Part model, mm, in its own coordinate system. Face numbers are marked on the shaded views. A direction names the side the tool comes from. Coordinates: 2 decimals unless noted, no trailing zeros. Write each loop counter-clockwise with the first axis right and the second up, starting at its lowest first coordinate (ties: lowest second). Pieces come first, ordered by that corner, then holes. Notation, with made-up numbers: M 24.5,-12.5 L 83.5,-12.5 A17 ccw 83.5,17.5 Z; hole C -23,22.25 d4. An arc over 180 degrees is marked long. Use a Markdown table: item, result. Add a question column.
Q1. Slice it at C-C on x = 0. Write the cut outline in (y, z), then the cut area to 3 significant figures.
Q2. Pin check, flat tips, straight feed: pin 1 Ø2.5 at (x, z) = (-2.5, -4) entering from +Y; pin 2 Ø2 at (y, z) = (20, 0) entering from -X; pin 3 Ø1 at (x, z) = (0.5, 0.5) entering from -Y; pin 4 Ø1.5 at (x, y) = (1, 17.5) entering from +Z. Stop position of each tip, or through.
Q3. Slice it at B-B on z = 0. Write the cut outline in (x, y).
Q4. Wall check: L1, parallel to Z at x = 1, y = 8.75; L2, parallel to Y at x = 1.5, z = -1.5; L3, parallel to Y at x = -2, z = 3.5. Give the ranges that are in metal, low to high. Write a range as from..to.
Q5. Slice it at D-D on y = 25. Write the cut outline in (x, z).
Q6. Tool access for the marked faces 1 and 2: list every direction of +Z, -Z, +X, -X, +Y, -Y with a clear straight run to the whole face (end or side of a thin tool).
Q7. Slice it at A-A on y = 4. Write the cut outline in (x, z), then the cut area to 3 significant figures.
Q8. Mould opens along Z. For the marked faces 3, 4, 5 and 6 say: released by +Z, released by -Z, zero draft, split by the parting line, or undercut.
Autodesk Inventor part; units mm, degrees
ref_plane "YZ Plane" through (0, 0, 0) normal (1, 0, 0) x (0, 1, 0)
ref_plane "XZ Plane" through (0, 0, 0) normal (0, 1, 0) x (-1, 0, 0)
ref_plane "XY Plane" through (0, 0, 0) normal (0, 0, 1) x (1, 0, 0)
sketch "Szkic1" plane through (0, 0, 0) normal (0, 1, 0) x (-1, 0, 0)
  line L0 (-2.75, 2.75) -> (2.75, 2.75)
  line L1 (2.75, 2.75) -> (2.75, -2.75)
  line L2 (2.75, -2.75) -> (-2.75, -2.75)
  line L3 (-2.75, -2.75) -> (-2.75, 2.75)
  line L4 (-2.75, 2.75) -> (2.75, -2.75) construction
  line L5 (2.75, 2.75) -> (-2.75, -2.75) construction
  line L6 (-2, 6) -> (2, 6)
  line L7 (6, 2) -> (6, -2)
  line L8 (2, -6) -> (-2, -6)
  line L9 (-6, -2) -> (-6, 2)
  line L10 (-6, 6) -> (6, -6) construction
  line L11 (6, 6) -> (-6, -6) construction
  arc A0 (6, 2) -> (2, 6) centre (2, 2) ccw
  arc A1 (2, -6) -> (6, -2) centre (2, -2) ccw
  arc A2 (-6, -2) -> (-2, -6) centre (-2, -2) ccw
  arc A3 (-2, 6) -> (-6, 2) centre (-2, 2) ccw
  point P0 (0, 0)
  dimension "d0" = 5.5
  dimension "d1" = 12
  dimension "d2" = 4
extrude "Wyciągnięcie proste1" add sketch "Szkic1" along normal blind 10
sketch "Szkic2" plane through (0, 10, 0) normal (0, 1, 0) x (1, 0, 0)
  arc A0 (-6, -2) -> (-2, -6) centre (-2, -2) ccw
  line L0 (-6, 2) -> (-6, -2)
  arc A1 (-2, 6) -> (-6, 2) centre (-2, 2) ccw
  line L1 (2, 6) -> (-2, 6)
  arc A2 (6, 2) -> (2, 6) centre (2, 2) ccw
  line L2 (6, -2) -> (6, 2)
  arc A3 (2, -6) -> (6, -2) centre (2, -2) ccw
  line L3 (-2, -6) -> (2, -6)
extrude "Wyciągnięcie proste2" add sketch "Szkic2" along normal blind 2
sketch "Szkic3" plane through (0, 12, 0) normal (0, 1, 0) x (1, 0, 0)
  circle A0 centre (0, 0) radius 4
  dimension "d7" = 8
extrude "Wyciągnięcie proste3" add sketch "Szkic3" along normal blind 15.45
sketch "Szkic5" plane through (0, 12, 0) normal (0, 1, 0) x (1, 0, 0)
  circle A0 centre (0, 0) radius 5.1
  dimension "d19" = 10.2
extrude "Wyciągnięcie proste4" add sketch "Szkic5" along normal blind 6.15
fillet "Zaokrąglenie2" radius 0.25 1 edges at (-4, 27.45, 0)
chamfer "Faza1" distance 1 angle 45 4 edges at (-2.75, 10, 0) (0, 10, 2.75) (2.75, 10, 0) (0, 10, -2.75)
sketch "Sketch6" plane through (0, 18.15, 0) normal (0, 1, 0) x (1, 0, 0)
  circle A0 centre (0, 0) radius 5.1
  circle A1 centre (0, 0) radius 4
extrude "Extrusion5" add sketch "Sketch6" along normal blind 3.3 contours A0 | A1
chamfer "Chamfer2" distance 1 angle 45 1 edges at (-5.1, 12, 0)
properties part number "CH_01_0020_servo_shaft_1"
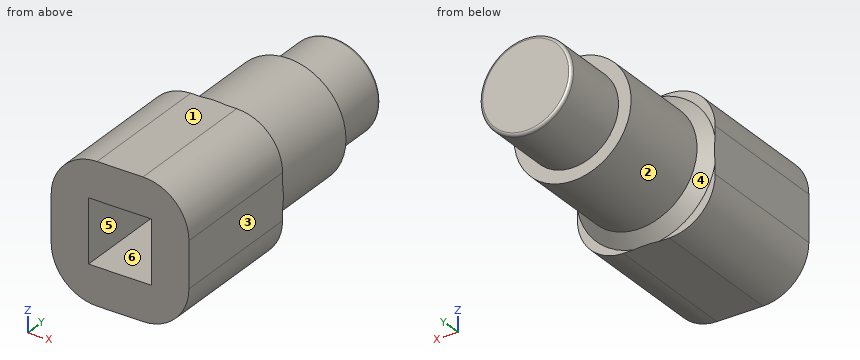
Recorded:
| question | item | result |
|---|---|---|
| 1 | outline | M 0,-6 L 12.1,-6 L 13,-5.1 L 21.45,-5.1 L 21.45,-4 L 27.2,-4 A0.25 ccw 27.45,-3.75 L 27.45,3.75 A0.25 ccw 27.2,4 L 21.45,4 L 21.45,5.1 L 13,5.1 L 12.1,6 L 0,6 L 0,2.75 L 9,2.75 L 10,1.75 L 10,-1.75 L 9,-2.75 L 0,-2.75 Z |
| 1 | area | 235 mm² |
| 2 | pin 1 | y = 27.45 |
| 2 | pin 2 | x = -5.1 |
| 2 | pin 3 | y = 10 |
| 2 | pin 4 | z = 5.09 |
| 3 | outline | M -6,0 L -2.75,0 L -2.75,9 L -1.75,10 L 1.75,10 L 2.75,9 L 2.75,0 L 6,0 L 6,12.1 L 5.1,13 L 5.1,21.45 L 4,21.45 L 4,27.2 A0.25 ccw 3.75,27.45 L -3.75,27.45 A0.25 ccw -4,27.2 L -4,21.45 L -5.1,21.45 L -5.1,13 L -6,12.1 Z |
| 4 | L1 | -6..-2.75, 2.75..6 |
| 4 | L2 | 10..27.45 |
| 4 | L3 | 0..21.45 |
| 5 | outline | C 0,0 d8 |
| 6 | face 1 | +Z, +X, -X, +Y, -Y |
| 6 | face 2 | +Y |
| 7 | outline | M -6,-2 A4 ccw -2,-6 L 2,-6 A4 ccw 6,-2 L 6,2 A4 ccw 2,6 L -2,6 A4 ccw -6,2 Z; hole M -2.75,-2.75 L 2.75,-2.75 L 2.75,2.75 L -2.75,2.75 Z |
| 7 | area | 100 mm² |
| 8 | face 3 | zero draft |
| 8 | face 4 | split by the parting line |
| 8 | face 5 | undercut |
| 8 | face 6 | undercut |
